Build history of the part. All positions in model axes, mm. Round coordinates to 2 decimals unless told otherwise and drop trailing zeros. Loops run counter-clockwise (first coordinate to the right, second up) from the corner with the lowest first, then second, coordinate; pieces in that order, holes last. Notation, with made-up numbers: (80, -13) -> (136, -13) arc R16 cw to (136, 10) -> close; hole circle Ø10 at (13.25, 31.5). An arc over 180 degrees is marked (long way). Put each result on its own line as item: value. Start each with the question number.
Item 1: Cut at B-B, the plane z = 0.3. Count the separate pieces of the cut face and the enclosed holes in it, plus the area to 3 significant figures.
Item 2: Cut at C-C, the plane y = 138.5. List the corners of the cut face in (x, z), plus the area to 3 significant figures.
Item 3: Flat gauge pins, fed straight in: pin 1 Ø1 at (x, y) = (115, 61.5) entering from -Z; pin 2 Ø2.5 at (x, y) = (190, 84.57) entering from +Z; pin 3 Ø0.6 at (x, z) = (251, 1) entering from -Y. Where does each tip first touch, or does it go through?
Item 4: Drill centre lines: probe 1 along Y at (x, z) = (65.5, 0.5); probe 2 along Y at (x, z) = (235, 1); probe 3 along Y at (x, z) = (190, 1.65). Where is each one in solid material? Low to high. Write a range as [from, to].
Item 5: Cut at A-A, the plane x = 204.5. List the corners of the cut face in (y, z), plus the area to 3 significant figures.
```python
from build123d import *

# Parameters (mm, degrees)
SKETCH1_W           = 250
SKETCH1_H           = 280.866666666
SKETCH1_R           = 2.3
SKETCH1_W_2         = 20
SKETCH1_H_2         = 2.2
BOSS_EXTRUDE1_DEPTH = 2
SKETCH2_W           = 2
SKETCH2_H           = 20
BOSS_EXTRUDE2_DEPTH = 2
SKETCH3_R           = 2.1
SKETCH3_W           = 28
SKETCH3_H           = 20
CUT_EXTRUDE1_DEPTH  = 5
SKETCH4_W           = 20
SKETCH4_H           = 30
CUT_EXTRUDE2_DEPTH  = 5
SKETCH5_R           = 2.1
CUT_EXTRUDE3_DEPTH  = 3
SKETCH6_R           = 2.1
CUT_EXTRUDE4_DEPTH  = 5
SKETCH7_R           = 2.1
CUT_EXTRUDE5_DEPTH  = 5


with BuildPart() as part:
    # Sketch1 → Boss-Extrude1 (new body)
    with BuildSketch(Plane.XY):
        with Locations((125, 135)):
            Rectangle(SKETCH1_W, SKETCH1_H)
        with Locations((125, 122.1)):
            Circle(SKETCH1_R, mode=Mode.SUBTRACT)
        with Locations((125, 202.1)):
            Circle(SKETCH1_R, mode=Mode.SUBTRACT)
        with Locations((190, 2.066666667)):
            Rectangle(SKETCH1_W_2, SKETCH1_H_2, mode=Mode.SUBTRACT)
        with Locations((60, 2.066666667)):
            Rectangle(SKETCH1_W_2, SKETCH1_H_2, mode=Mode.SUBTRACT)
        with Locations((190, 267.933333333)):
            Rectangle(SKETCH1_W_2, SKETCH1_H_2, mode=Mode.SUBTRACT)
        with Locations((60, 267.933333333)):
            Rectangle(SKETCH1_W_2, SKETCH1_H_2, mode=Mode.SUBTRACT)
    extrude(amount=BOSS_EXTRUDE1_DEPTH)

    # Sketch2 → Boss-Extrude2 (add)
    with BuildSketch(Plane.XY.offset(2)):
        with Locations((-1, 195.433333333)):
            Rectangle(SKETCH2_W, SKETCH2_H)
        with Locations((-1, 74.566666667)):
            Rectangle(SKETCH2_W, SKETCH2_H)
        with Locations((251, 195.433333333)):
            Rectangle(SKETCH2_W, SKETCH2_H)
        with Locations((251, 74.566666667)):
            Rectangle(SKETCH2_W, SKETCH2_H)
    extrude(amount=-BOSS_EXTRUDE2_DEPTH)

    # Sketch3 → Cut-Extrude1 (cut)
    with BuildSketch(Plane.XY.offset(2)):
        with Locations((190, 84.566666667)):
            Circle(SKETCH3_R)
        with Locations((230, 84.566666667)):
            Circle(SKETCH3_R)
        with Locations((210, 84.566666667)):
            Rectangle(SKETCH3_W, SKETCH3_H)
    extrude(amount=-CUT_EXTRUDE1_DEPTH, mode=Mode.SUBTRACT)

    # Sketch4 → Cut-Extrude2 (cut)
    with BuildSketch(Plane.XY.offset(2)):
        with Locations((86.25, 34.766666667)):
            Rectangle(SKETCH4_W, SKETCH4_H)
    extrude(amount=-CUT_EXTRUDE2_DEPTH, mode=Mode.SUBTRACT)

    # Sketch5 → Cut-Extrude3 (cut, through all)
    with BuildSketch(Plane.XY.offset(2)):
        with Locations((98.18627451, 12.72)):
            Circle(SKETCH5_R)
        with Locations((74.31372549, 12.72)):
            Circle(SKETCH5_R)
        with Locations((74.31372549, 51.68)):
            Circle(SKETCH5_R)
        with Locations((98.18627451, 51.68)):
            Circle(SKETCH5_R)
    extrude(amount=-CUT_EXTRUDE3_DEPTH, mode=Mode.SUBTRACT)

    # Sketch6 → Cut-Extrude4 (cut)
    with BuildSketch(Plane.XY.offset(2)):
        with Locations((235, 250)):
            Circle(SKETCH6_R)
        with Locations((15, 250)):
            Circle(SKETCH6_R)
    extrude(amount=-CUT_EXTRUDE4_DEPTH, mode=Mode.SUBTRACT)

    # Sketch7 → Cut-Extrude5 (cut)
    with BuildSketch(Plane.XY.offset(2)):
        with Locations((15, 104.566666667)):
            Circle(SKETCH7_R)
        with Locations((235, 104.566666667)):
            Circle(SKETCH7_R)
    extrude(amount=-CUT_EXTRUDE5_DEPTH, mode=Mode.SUBTRACT)


solid = part.part
```
Reply:
1. separate pieces: 1
1. enclosed holes: 18
1. area: 68,900 mm^2
2. outline: (0, 0) -> (250, 0) -> (250, 2) -> (0, 2) -> close
2. area: 500 mm^2
3. pin 1: stops at z = 0
3. pin 2: passes through
3. pin 3: stops at y = 64.57
4. probe 1: y = [-5.43, 0.97], [3.17, 266.83], [269.03, 275.43]
4. probe 2: y = [-5.43, 102.47], [106.67, 247.9], [252.1, 275.43]
4. probe 3: y = [-5.43, 0.97], [3.17, 82.47], [86.67, 266.83], [269.03, 275.43]
5. outline: (-5.43, 0) -> (74.57, 0) -> (74.57, 2) -> (-5.43, 2) -> close; (94.57, 0) -> (275.43, 0) -> (275.43, 2) -> (94.57, 2) -> close
5. area: 522 mm^2
